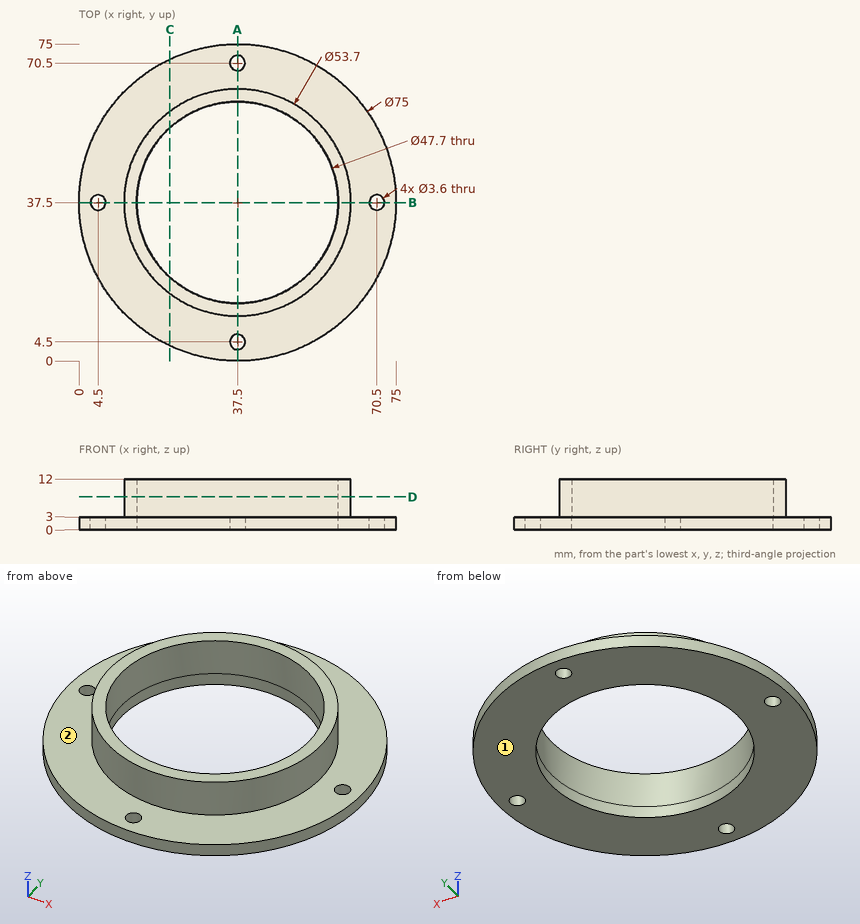
Input: dimensioned drawing with shaded views. Units: mm. Origin: part minimum x, y, z. A direction names the side the tool comes from. Coordinates: 2 decimals unless noted, no trailing zeros. Loops run counter-clockwise (first coordinate to the right, second up) from the corner with the lowest first, then second, coordinate; pieces in that order, holes last. Notation, with made-up numbers: M -2.5,51.25 L 29.5,51.25 A24 cw 29.5,85.25 Z; hole C 1,-13 d10. An arc over 180 degrees is marked long. Use a Markdown table: item, result. Add a question column.
Q1. First-contact query: pin 1 (4 mm diameter, centred on x = 4.5, y = 37.5, fed in from -Z); pin 2 (4 mm diameter, centred on y = 13.5, z = 9.5, fed in from +X); pin 3 (5 mm diameter, centred on y = 35.5, z = 5, fed in from -X); pin 4 (1.5 mm diameter, centred on x = 63.5, z = 2.5, fed in from -Y). Flat tips, straight axial feed; report the tip coordinate or a pass-through.
Q2. Section query D-D, the plane z = 7.75. Return loops of the section in (x, y), and give its area (3 significant figures).
Q3. Access query for the marked faces 1 and 2. Directions: +Z, -Z, +X, -X, +Y, -Y. A direction counts if a zero-diameter tool reaches every point of the face in a straight line with its end or side. Return the directions, or none.
Q4. Section query C-C, the plane x = 21.5. Return loops of the section in (y, z), and give its area (3 significant figures).
Q5. Material intervals for L1, parallel to Y at x = 37.5, z = 1.5; L2, parallel to Y at x = 37.5, z = 10; L3, parallel to Z at x = 46, y = 63, sorted ascending.
Q6. Section query A-A, the plane x = 37.5. Return loops of the section in (y, z), and give its area (3 significant figures).
Result:
| question | item | result |
|---|---|---|
| 1 | pin 1 | stops at z = 0 |
| 1 | pin 2 | stops at x = 52.89 |
| 1 | pin 3 | stops at x = 0 |
| 1 | pin 4 | stops at y = 9.77 |
| 2 | outline | C 37.5,37.5 d53.7; hole C 37.5,37.5 d47.7 |
| 2 | area | 478 mm2 |
| 3 | face 1 | -Z, +X, -X, +Y, -Y |
| 3 | face 2 | +Z |
| 4 | outline | M 3.58,0 L 19.81,0 L 19.81,12 L 15.94,12 L 15.94,3 L 3.58,3 Z; M 55.19,0 L 71.42,0 L 71.42,3 L 59.06,3 L 59.06,12 L 55.19,12 Z |
| 4 | area | 167 mm2 |
| 5 | L1 | y = 0 to 2.7, 6.3 to 13.65, 61.35 to 68.7, 72.3 to 75 |
| 5 | L2 | y = 10.65 to 13.65, 61.35 to 64.35 |
| 5 | L3 | z = 0 to 3 |
| 6 | outline | M 0,0 L 2.7,0 L 2.7,3 L 0,3 Z; M 6.3,0 L 13.65,0 L 13.65,12 L 10.65,12 L 10.65,3 L 6.3,3 Z; M 61.35,0 L 68.7,0 L 68.7,3 L 64.35,3 L 64.35,12 L 61.35,12 Z; M 72.3,0 L 75,0 L 75,3 L 72.3,3 Z |
| 6 | area | 114 mm2 |
